from build123d import *

# Parameters (mm, degrees)
BOSS_EXTRUDE1_DEPTH      = 3.175
SKETCH2_R                = 11.5
CUT_EXTRUDE1_DEPTH       = 4.175
M3_CLEARANCE_HOLE1_D     = 3.4
M3_CLEARANCE_HOLE1_DEPTH = 3.175


with BuildPart() as part:
    # Sketch1 → Boss-Extrude1 (new body)
    with BuildSketch(Plane.XY):
        Polygon((-17, -21.15), (17, -21.15), (21.15, -17), (21.15, 17), (17, 21.15), (-17, 21.15), (-21.15, 17), (-21.15, -17), align=None)
    extrude(amount=BOSS_EXTRUDE1_DEPTH)

    # Sketch2 → Cut-Extrude1 (cut, through all)
    with BuildSketch(Plane.XY.offset(3.175)):
        Circle(SKETCH2_R)
    extrude(amount=-CUT_EXTRUDE1_DEPTH, mode=Mode.SUBTRACT)

    # M3 Clearance Hole1
    with Locations(Plane.XY.offset(3.175)):
        with Locations((-15.5, 15.5), (15.5, 15.5), (15.5, -15.5), (-15.5, -15.5)):
            Hole(M3_CLEARANCE_HOLE1_D / 2, depth=M3_CLEARANCE_HOLE1_DEPTH)


solid = part.part
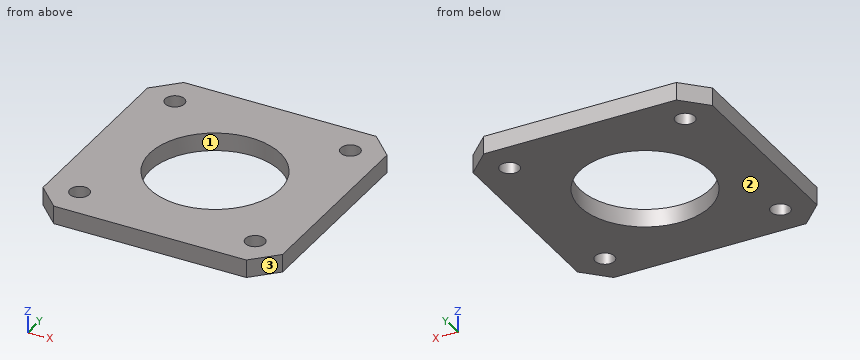
Source: CAD feature listing. Evaluate the final solid. Frame: model axes, mm. Face numbers are marked on the shaded views. Round coordinates to 2 decimals unless told otherwise and drop trailing zeros. Write each loop counter-clockwise with the first axis right and the second up, starting at its lowest first coordinate (ties: lowest second). Pieces come first, ordered by that corner, then holes. Notation, with made-up numbers: (-11.5, -11) - (9.5, -11) arc R34 cw to (9.5, 23) - close; hole circle Ø1 at (-2.75, -29.5). An arc over 180 degrees is marked (long way). Use CSV: the item, a comma, the result in double quotes. Start each with the question number.
(1) Mould query, pull axis Y, two halves, no side actions, for the marked faces 1, 2 and 3. Classes: pulls with the +Y half, pulls with the -Y half, needs draft (parallel to the pull), parting line crosses it, or undercut.
(2) Cut plane B-B, the plane z = 0.6. Return loops of the section in (x, y).
(3) Material intervals for probe 1 along Y at (x, z) = (-15.5, 1.45); probe 2 along X at (y, z) = (15, 1); probe 3 along X at (y, z) = (14, 0.3), sorted ascending. Write a range as [from, to].
(4) Cut plane A-A, the plane y = 0. Return loops of the section in (x, z) (3 decimals), and give its area (3 significant figures).
(5) Cut plane D-D, the plane y = 15.5. Return loops of the section in (x, z) (3 decimals).
(6) First-contact query: pin 1 Ø20.5 at (x, y) = (0, 0) entering from +Z. Flat tip, straight axial feed; report the tip coordinate or a pass-through.
Geometry says:
1,face 1,"undercut"
1,face 2,"needs draft"
1,face 3,"pulls with the -Y half"
2,outline,"(-21.15, -17) - (-17, -21.15) - (17, -21.15) - (21.15, -17) - (21.15, 17) - (17, 21.15) - (-17, 21.15) - (-21.15, 17) - close; hole circle Ø3.4 at (-15.5, -15.5); hole circle Ø3.4 at (-15.5, 15.5); hole circle Ø23 at (0, 0); hole circle Ø3.4 at (15.5, -15.5); hole circle Ø3.4 at (15.5, 15.5)"
3,probe 1,"[-21.15, -17.2], [-13.8, 13.8], [17.2, 21.15]"
3,probe 2,"[-21.15, -17.12], [-13.88, 13.88], [17.12, 21.15]"
3,probe 3,"[-21.15, -16.3], [-14.7, 14.7], [16.3, 21.15]"
4,outline,"(-21.15, 0) - (-11.5, 0) - (-11.5, 3.175) - (-21.15, 3.175) - close; (11.5, 0) - (21.15, 0) - (21.15, 3.175) - (11.5, 3.175) - close"
4,area,"61.3 mm²"
5,outline,"(-21.15, 0) - (-17.2, 0) - (-17.2, 3.175) - (-21.15, 3.175) - close; (-13.8, 0) - (13.8, 0) - (13.8, 3.175) - (-13.8, 3.175) - close; (17.2, 0) - (21.15, 0) - (21.15, 3.175) - (17.2, 3.175) - close"
6,pin 1,"through"
